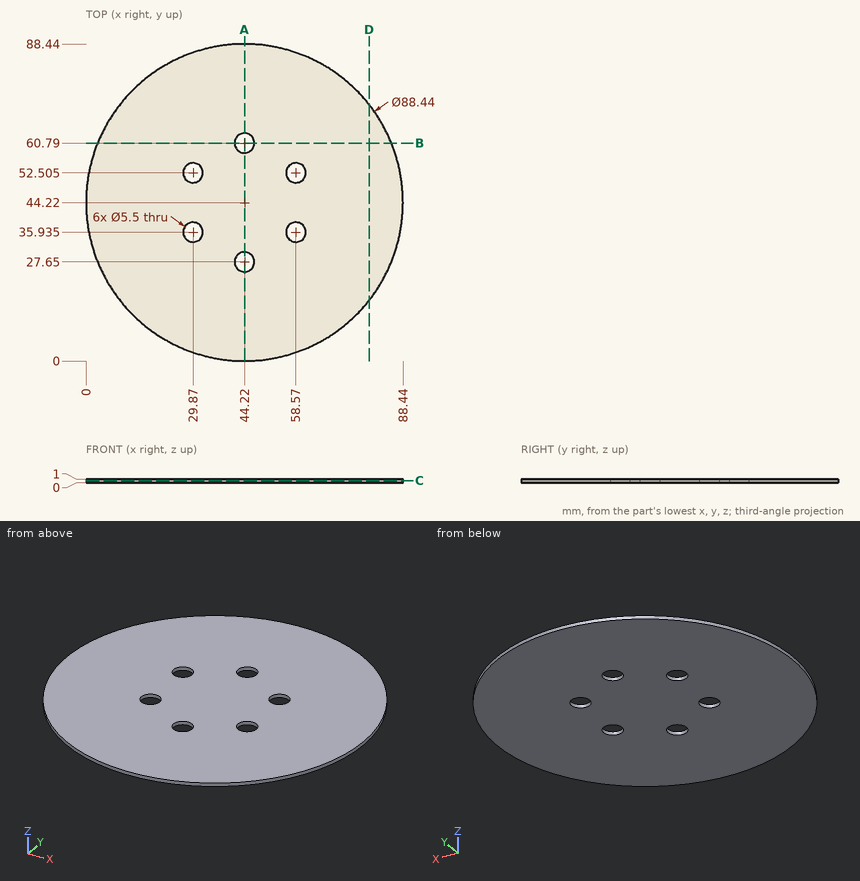
Part print with two shaded views. Sizes in mm from the minimum x, y, z corner. Round coordinates to 2 decimals unless told otherwise and drop trailing zeros. Loops run counter-clockwise (first coordinate to the right, second up) from the corner with the lowest first, then second, coordinate; pieces in that order, holes last.
Item 1: Saw through at D-D (x = 79). List the corners of the cut face in (y, z), then the cut area to 3 significant figures.
Item 2: Drill centre lines: line 1 along Y through (x, z) = (57, 0.35); line 2 along X through (y, z) = (63, 0.6); line 3 along X through (y, z) = (27, 0.75). Where is each one in solid material? Low to high.
Item 3: Saw through at B-B (y = 60.79). List the corners of the cut face in (x, z).
Item 4: Saw through at A-A (x = 44.22). List the corners of the cut face in (y, z).
Item 5: Saw through at C-C (z = 0.55). List the corners of the cut face in (x, y) (3 decimals), then the cut area to 3 significant figures.
Worked answers:
1. outline: (16.91, 0) - (71.53, 0) - (71.53, 1) - (16.91, 1) - close
1. area: 54.6 mm2
2. line 1: y = 1.89 to 33.68, 38.19 to 50.25, 54.76 to 86.55
2. line 2: x = 4.19 to 42.58, 45.86 to 84.25
2. line 3: x = 3.49 to 41.55, 46.89 to 84.95
3. outline: (3.22, 0) - (41.47, 0) - (41.47, 1) - (3.22, 1) - close; (46.97, 0) - (85.22, 0) - (85.22, 1) - (46.97, 1) - close
4. outline: (0, 0) - (24.9, 0) - (24.9, 1) - (0, 1) - close; (30.4, 0) - (58.04, 0) - (58.04, 1) - (30.4, 1) - close; (63.54, 0) - (88.44, 0) - (88.44, 1) - (63.54, 1) - close
5. outline: circle Ø88.44 at (44.22, 44.22); hole circle Ø5.5 at (29.87, 35.935); hole circle Ø5.5 at (29.87, 52.505); hole circle Ø5.5 at (44.22, 27.65); hole circle Ø5.5 at (44.22, 60.79); hole circle Ø5.5 at (58.57, 35.935); hole circle Ø5.5 at (58.57, 52.505)
5. area: 6,000 mm2
